Geometry check sheet. Reference: the model listing, model coordinates, mm. Face numbers are marked on the shaded views. A direction names the side the tool comes from. Round coordinates to 2 decimals unless told otherwise and drop trailing zeros. Write each loop counter-clockwise with the first axis right and the second up, starting at its lowest first coordinate (ties: lowest second). Pieces come first, ordered by that corner, then holes.
Item 1: Cross-section at B-B (x = -13). Enter the section's corners in (y, z), then the cut area to 3 significant figures.
Item 2: Cross-section at D-D (z = -14). Enter the section's corners in (x, y), then the cut area to 3 significant figures.
Item 3: Cross-section at C-C (z = 30). Enter the section's corners in (x, y).
Item 4: Cross-section at A-A (y = -33). State how many separate pieces and enclosed holes the cut face has, then the cut area to 3 significant figures.
Item 5: Access from +Z, -Z, +X, -X, +Y, -Y to the whole of each face (thin tool, end or side, straight path). Record for the marked faces 5 and 6.
Item 6: Draft check along Z on the marked faces 1, 2, 3 and 4. Enter one of: pulls with the +Z half, pulls with the -Z half, needs draft (parallel to the pull), parting line crosses it, or undercut.
Item 7: Scan lines: probe 1 along X at (y, z) = (-24, -35); probe 2 along X at (y, z) = (-31, -16.5); probe 3 along Z at (x, y) = (-27, -28.5). Record each from-to range of solid material in increasing order.
Item 8: Depth check by flat-ended pin: P1, Ø12, axis at x = -32.5, z = 38.5, coming from the -Y side; P2, Ø3, axis at x = -40.5, z = -35.5, coming from the -Y side; P3, Ø2, axis at x = -14, y = -23.5, coming from the -Z side. Enter the tip coordinate at first touch or a pass-through.
from build123d import *

# Parameters (mm, degrees)
BOSS_EXTRUDE1_DEPTH      = 1
BOSS_EXTRUDE1_DEPTH_BACK = 3
SKETCH1_W                = 110
SKETCH1_H                = 100
SKETCH2_W                = 110
SKETCH2_H                = 100
SKETCH2_W_2              = 104
SKETCH2_H_2              = 94
BOSS_EXTRUDE2_DEPTH      = 35
SKETCH3_R                = 3
SKETCH3_R_2              = 1.3
BOSS_EXTRUDE3_DEPTH      = 32
SKETCH5_W                = 12
SKETCH5_H                = 20
CUT_EXTRUDE5_DEPTH       = 32
SKETCH6_W                = 15
SKETCH6_H                = 10
CUT_EXTRUDE6_DEPTH       = 32
SKETCH7_R                = 8
CUT_EXTRUDE7_DEPTH       = 22
SKETCH8_W                = 12
SKETCH8_H                = 10
CUT_EXTRUDE8_DEPTH       = 22
SKETCH9_W                = 5
SKETCH9_H                = 50
CUT_EXTRUDE9_DEPTH       = 10
FILLET1_R                = 2
FILLET2_R                = 3
FILLET3_R                = 4


with BuildPart() as part:
    # Sketch1 → Boss-Extrude1 (new, two sides: drawn at the far end of the back side and taken through both)
    with BuildSketch(Plane(origin=(0, 0, 0), x_dir=(1, 0, 0), z_dir=(0, 1, 0)).offset(-BOSS_EXTRUDE1_DEPTH_BACK)):
        Rectangle(SKETCH1_W, SKETCH1_H)
    extrude(amount=BOSS_EXTRUDE1_DEPTH + BOSS_EXTRUDE1_DEPTH_BACK)

    # Sketch2 → Boss-Extrude2 (add)
    with BuildSketch(Plane.XZ.offset(3)):
        Rectangle(SKETCH2_W, SKETCH2_H)
        Rectangle(SKETCH2_W_2, SKETCH2_H_2, mode=Mode.SUBTRACT)
    extrude(amount=BOSS_EXTRUDE2_DEPTH)

    # Sketch3 → Boss-Extrude3 (add)
    # profile 1 of 4: a face of its own
    with BuildSketch(Plane.XZ.offset(3)):
        with Locations(Location((-41, 35, 0), (0, 0, 90))):
            Circle(SKETCH3_R)
        with Locations(Location((-41, 35, 0), (0, 0, 270))):
            Circle(SKETCH3_R_2, mode=Mode.SUBTRACT)
    # profile 2 of 4: a face of its own
    with BuildSketch(Plane.XZ.offset(3)):
        with Locations(Location((-41, -35, 0), (0, 0, 90))):
            Circle(SKETCH3_R)
        with Locations(Location((-41, -35, 0), (0, 0, 90))):
            Circle(SKETCH3_R_2, mode=Mode.SUBTRACT)
    # profile 3 of 4: a face of its own
    with BuildSketch(Plane.XZ.offset(3)):
        with Locations(Location((41, -35, 0), (0, 0, 90))):
            Circle(SKETCH3_R)
        with Locations(Location((41, -35, 0), (0, 0, 270))):
            Circle(SKETCH3_R_2, mode=Mode.SUBTRACT)
    # profile 4 of 4: a face of its own
    with BuildSketch(Plane.XZ.offset(3)):
        with Locations(Location((41, 35, 0), (0, 0, 90))):
            Circle(SKETCH3_R)
        with Locations(Location((41, 35, 0), (0, 0, 90))):
            Circle(SKETCH3_R_2, mode=Mode.SUBTRACT)
    extrude(amount=BOSS_EXTRUDE3_DEPTH)

    # Sketch5 → Cut-Extrude5 (cut)
    with BuildSketch(Plane(origin=(0, 0, -50), x_dir=(-1, 0, 0), z_dir=(0, 0, -1))):
        with Locations((-28, -28)):
            Rectangle(SKETCH5_W, SKETCH5_H)
        with Locations((14, -28)):
            Rectangle(SKETCH5_W, SKETCH5_H)
    extrude(amount=-CUT_EXTRUDE5_DEPTH, mode=Mode.SUBTRACT)

    # Sketch6 → Cut-Extrude6 (cut)
    with BuildSketch(Plane.XY.offset(50)):
        with Locations((-23, -23)):
            Rectangle(SKETCH6_W, SKETCH6_H)
    extrude(amount=-CUT_EXTRUDE6_DEPTH, mode=Mode.SUBTRACT)

    # Sketch7 → Cut-Extrude7 (cut)
    with BuildSketch(Plane(origin=(55, 0, 0), x_dir=(0, 0, -1), z_dir=(1, 0, 0))):
        with Locations((-11, -20.5)):
            Circle(SKETCH7_R)
        with Locations((14, -20.5)):
            Circle(SKETCH7_R)
    extrude(amount=-CUT_EXTRUDE7_DEPTH, mode=Mode.SUBTRACT)

    # Sketch8 → Cut-Extrude8 (cut)
    with BuildSketch(Plane(origin=(0, 1, 0), x_dir=(1, 0, 0), z_dir=(0, 1, 0))):
        with Locations((28, 33)):
            Rectangle(SKETCH8_W, SKETCH8_H)
        with Locations((-14, 33)):
            Rectangle(SKETCH8_W, SKETCH8_H)
    extrude(amount=-CUT_EXTRUDE8_DEPTH, mode=Mode.SUBTRACT)

    # Sketch9 → Cut-Extrude9 (cut)
    with BuildSketch(Plane(origin=(0, 1, 0), x_dir=(1, 0, 0), z_dir=(0, 1, 0))):
        with Locations((-35, -15)):
            Rectangle(SKETCH9_W, SKETCH9_H)
        with Locations((-20, -15)):
            Rectangle(SKETCH9_W, SKETCH9_H)
        with Locations((-5, -15)):
            Rectangle(SKETCH9_W, SKETCH9_H)
        with Locations((10, -15)):
            Rectangle(SKETCH9_W, SKETCH9_H)
        with Locations((25, -15)):
            Rectangle(SKETCH9_W, SKETCH9_H)
    extrude(amount=-CUT_EXTRUDE9_DEPTH, mode=Mode.SUBTRACT)

    # Fillet1
    fillet1_edges = [part.edges().sort_by_distance(p)[0] for p in [
        (-32.5, -1, -10),
        (-32.5, -1, 40),
        (-37.5, -1, 40),
        (-37.5, -1, -10),
        (-17.5, -1, -10),
        (-17.5, -1, 40),
        (-22.5, -1, 40),
        (-22.5, -1, -10),
        (-2.5, -1, -10),
        (-2.5, -1, 40),
        (-7.5, -1, 40),
        (-7.5, -1, -10),
        (7.5, -1, 40),
        (7.5, -1, -10),
        (12.5, -1, -10),
        (12.5, -1, 40),
        (22.5, -1, 40),
        (22.5, -1, -10),
        (27.5, -1, -10),
        (27.5, -1, 40),
    ]]
    fillet(fillet1_edges, radius=FILLET1_R)

    # Fillet2
    fillet2_edges = [part.edges().sort_by_distance(p)[0] for p in [
        (-20, -18, -48.5),
        (-8, -18, -48.5),
        (34, -18, -48.5),
        (22, -18, -48.5),
    ]]
    fillet(fillet2_edges, radius=FILLET2_R)

    # Fillet3
    fillet3_edges = [part.edges().sort_by_distance(p)[0] for p in [
        (-15.5, -18, 48.5),
        (-15.5, -28, 48.5),
        (-30.5, -28, 48.5),
        (-30.5, -18, 48.5),
    ]]
    fillet(fillet3_edges, radius=FILLET3_R)


solid = part.part
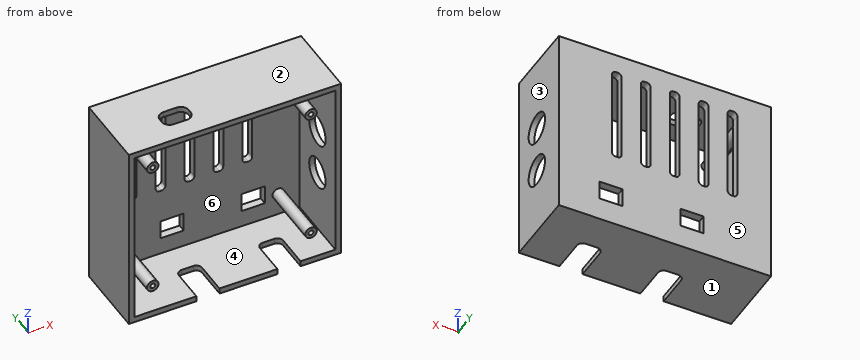
Resolved:
1. outline: (-38, 47) - (-3, 47) - (-3, -28) - (1, -28) - (1, 50) - (-38, 50) - close; (-18, -50) - (1, -50) - (1, -38) - (-3, -38) - (-3, -47) - (-18, -47) - close
1. area: 510 mm2
2. outline: (-55, -38) - (-52, -38) - (-52, -3) - (52, -3) - (52, -12.5) - (55, -12.5) - (55, 1) - (-55, 1) - close; (52, -38) - (55, -38) - (55, -28.5) - (52, -28.5) - close
2. area: 602 mm2
3. outline: (-55, -38) - (-52, -38) - (-52, -3) - (-37.5, -3) - (-37.5, 1) - (-55, 1) - close; (-32.5, -3) - (-22.5, -3) - (-22.5, 1) - (-32.5, 1) - close; (-17.5, -3) - (-7.5, -3) - (-7.5, 1) - (-17.5, 1) - close; (-2.5, -3) - (7.5, -3) - (7.5, 1) - (-2.5, 1) - close; (12.5, -3) - (22.5, -3) - (22.5, 1) - (12.5, 1) - close; (27.5, -3) - (52, -3) - (52, -38) - (55, -38) - (55, 1) - (27.5, 1) - close
4. separate pieces: 6
4. enclosed holes: 4
4. area: 1,240 mm2
5. face 5: +Z, -Z, +X, -X, +Y
5. face 6: -Y
6. face 1: pulls with the -Z half
6. face 2: pulls with the +Z half
6. face 3: needs draft
6. face 4: undercut
7. probe 1: x = -55 to -52, -44 to -42.3, -39.7 to -38, 38 to 39.7, 42.3 to 44, 52 to 55
7. probe 2: x = -55 to -52, 52 to 55
7. probe 3: z = -50 to -47, 47 to 50
8. P1: stops at y = -3
8. P2: stops at y = -35
8. P3: stops at z = 47
